Could you check a few things on this model? Use its own coordinates, in mm. A direction names the side the tool comes from. Coordinates: 2 decimals unless noted, no trailing zeros. Loops run counter-clockwise (first coordinate to the right, second up) from the corner with the lowest first, then second, coordinate; pieces in that order, holes last.
from build123d import *

# Parameters (mm, degrees)
SKETCH_2_R          = 1.5
EXTRUDE_1_DEPTH     = 52
CUT_EXTRUDE_START   = -3
SKETCH_3_R          = 19
SKETCH_3_R_2        = 1.6
CUT_EXTRUDE_1_DEPTH = 25
SKETCH_3_3_R        = 1.6
CUT_EXTRUDE_2_DEPTH = 25
SKETCH_5_R          = 17.6
CUT_EXTRUDE_3_DEPTH = 310.300460798
SKETCH_6_R          = 6.1
CUT_EXTRUDE_4_DEPTH = 3
CUT_EXTRUDE_5_REACH = 313.3
SKETCH_7_W          = 42
SKETCH_7_H          = 28
CHAMFER_1_SIZE      = 5
CHAMFER_5_SIZE      = 10
CHAMFER_5_SIZE2     = 5.773502692
EXTRUDE_2_DEPTH     = 2


with BuildPart() as part:
    # 草图2 → 凸台-拉伸1 (new body)
    with BuildSketch(Plane(origin=(0, 0, 255.313805399), x_dir=(-1, 0, 0), z_dir=(0, 0, -1))):
        Polygon((21, 18), (19, 20), (-19, 20), (-21, 18), (-21, -25), (21, -25), align=None)
        with Locations((16, -15)):
            Circle(SKETCH_2_R, mode=Mode.SUBTRACT)
        with Locations((16, 15)):
            Circle(SKETCH_2_R, mode=Mode.SUBTRACT)
        with Locations((-16, 15)):
            Circle(SKETCH_2_R, mode=Mode.SUBTRACT)
        with Locations((-16, -15)):
            Circle(SKETCH_2_R, mode=Mode.SUBTRACT)
    extrude(amount=-EXTRUDE_1_DEPTH)

    # 草图3 → 切除-拉伸1 (cut)
    # profile 1 of 7: a face of its own
    with BuildSketch(Plane.XZ.offset(25).offset(CUT_EXTRUDE_START)):
        with Locations(Location((0, 279.313805399, 0), (0, 0, 270))):
            Circle(SKETCH_3_R)
        with Locations((15.5, 279.313805399)):
            Circle(SKETCH_3_R_2, mode=Mode.SUBTRACT)
        with Locations((7.75, 292.737199157)):
            Circle(SKETCH_3_R_2, mode=Mode.SUBTRACT)
        with Locations((-7.75, 292.737199157)):
            Circle(SKETCH_3_R_2, mode=Mode.SUBTRACT)
        with Locations((-15.5, 279.313805399)):
            Circle(SKETCH_3_R_2, mode=Mode.SUBTRACT)
        with Locations((-7.75, 265.89041164)):
            Circle(SKETCH_3_R_2, mode=Mode.SUBTRACT)
        with Locations((7.75, 265.89041164)):
            Circle(SKETCH_3_R_2, mode=Mode.SUBTRACT)
    # profile 2 of 7: a face of its own
    with BuildSketch(Plane.XZ.offset(25).offset(CUT_EXTRUDE_START)):
        with Locations((7.75, 292.737199157)):
            Circle(SKETCH_3_R_2)
    # profile 3 of 7: a face of its own
    with BuildSketch(Plane.XZ.offset(25).offset(CUT_EXTRUDE_START)):
        with Locations((-7.75, 292.737199157)):
            Circle(SKETCH_3_R_2)
    # profile 4 of 7: a face of its own
    with BuildSketch(Plane.XZ.offset(25).offset(CUT_EXTRUDE_START)):
        with Locations((-15.5, 279.313805399)):
            Circle(SKETCH_3_R_2)
    # profile 5 of 7: a face of its own
    with BuildSketch(Plane.XZ.offset(25).offset(CUT_EXTRUDE_START)):
        with Locations((-7.75, 265.89041164)):
            Circle(SKETCH_3_R_2)
    # profile 6 of 7: a face of its own
    with BuildSketch(Plane.XZ.offset(25).offset(CUT_EXTRUDE_START)):
        with Locations((7.75, 265.89041164)):
            Circle(SKETCH_3_R_2)
    # profile 7 of 7: a face of its own
    with BuildSketch(Plane.XZ.offset(25).offset(CUT_EXTRUDE_START)):
        with Locations((15.5, 279.313805399)):
            Circle(SKETCH_3_R_2)
    extrude(amount=-CUT_EXTRUDE_1_DEPTH, mode=Mode.SUBTRACT)

    # 草图3<3> → 切除-拉伸2 (cut)
    with BuildSketch(Plane.XZ.offset(25)):
        with Locations(Location((-7.75, 292.737199157, 0), (0, 0, 270))):
            Circle(SKETCH_3_3_R)
        with Locations(Location((7.75, 292.737199157, 0), (0, 0, 270))):
            Circle(SKETCH_3_3_R)
        with Locations(Location((-15.5, 279.313805399, 0), (0, 0, 270))):
            Circle(SKETCH_3_3_R)
        with Locations(Location((-7.75, 265.89041164, 0), (0, 0, 270))):
            Circle(SKETCH_3_3_R)
        with Locations(Location((7.75, 265.89041164, 0), (0, 0, 270))):
            Circle(SKETCH_3_3_R)
        with Locations(Location((15.5, 279.313805399, 0), (0, 0, 270))):
            Circle(SKETCH_3_3_R)
    extrude(amount=-CUT_EXTRUDE_2_DEPTH, mode=Mode.SUBTRACT)

    # 草图5 → 切除-拉伸3 (cut, through all)
    with BuildSketch(Plane.XZ.offset(-3)):
        with Locations(Location((0, 279.313805399, 0), (0, 0, 270))):
            Circle(SKETCH_5_R)
    extrude(amount=-CUT_EXTRUDE_3_DEPTH, mode=Mode.SUBTRACT)

    # 草图6 → 切除-拉伸4 (cut)
    with BuildSketch(Plane.XZ.offset(25)):
        with Locations(Location((0, 286.313805399, 0), (0, 0, 270))):
            Circle(SKETCH_6_R)
    extrude(amount=-CUT_EXTRUDE_4_DEPTH, mode=Mode.SUBTRACT)

    # 切除-拉伸5: up to this face of the body (flat: up to its plane)
    cut_extrude_5_end = Plane(part.part.faces().sort_by_distance((0, -22, 278.469302594))[0])
    # 草图7 → 切除-拉伸5 (cut, up to the picked face)
    with BuildSketch(Plane(origin=(0, 20, 0), x_dir=(1, 0, 0), z_dir=(0, 1, 0)), mode=Mode.PRIVATE) as cut_extrude_5_sk1:
        with Locations((0, -293.313805399)):
            Rectangle(SKETCH_7_W, SKETCH_7_H)
    cut_extrude_5_tool1 = split(extrude(cut_extrude_5_sk1.sketch, amount=-CUT_EXTRUDE_5_REACH, mode=Mode.PRIVATE), bisect_by=cut_extrude_5_end, keep=Keep.BOTH, mode=Mode.PRIVATE)
    add(cut_extrude_5_tool1.solids().sort_by(Axis((0, 20, 293.313805), (0, -1, 0)))[0], mode=Mode.SUBTRACT)

    # 倒角1
    chamfer_1_edges = [part.edges().sort_by_distance(p)[0] for p in [
        (21, -23.5, 307.313805399),
        (-21, -23.5, 307.313805399),
    ]]
    chamfer(chamfer_1_edges, length=CHAMFER_1_SIZE)

    # 倒角5
    chamfer_5_edges = [part.edges().sort_by_distance(p)[0] for p in [
        (-18.3, 20, 279.313805399),
        (18.3, 20, 279.313805399),
    ]]
    chamfer_5_side = [part.faces().sort_by_distance(p)[0] for p in [
        (0, 20, 255.7632495),
    ]]
    chamfer(chamfer_5_edges, length=CHAMFER_5_SIZE, length2=CHAMFER_5_SIZE2, reference=chamfer_5_side[0])

    # 草图8 → 凸台-拉伸2 (add)
    with BuildSketch(Plane(origin=(21, 0, 0), x_dir=(0, 0, -1), z_dir=(1, 0, 0))):
        Polygon((-279.313805399, -22), (-279.313805399, 2.989978389), (-290.216930942, -22), align=None)
    extrude_2 = extrude(amount=-EXTRUDE_2_DEPTH)

    # 镜向1: 凸台-拉伸2 across plane
    add(extrude_2.mirror(Plane(origin=(0, 0, 0), x_dir=(0, 0, 1), z_dir=(1, 0, 0))))


solid = part.part
(1) Imagine slicing it at C-C, the plane y = 12.5. Write out the boundary of the cut face in (x, z), and give its area (3 significant figures).
Answers:
outline: (-21, 255.31) - (21, 255.31) - (21, 279.31) - (17.6, 279.31) arc R17.6 cw to (-17.6, 279.31) - (-21, 279.31) - close
area: 521 mm2
(2) I need wall thicknesses on probe 1 along X at (y, z) = (-12, 280.5); probe 2 along X at (y, z) = (-14, 258); probe 3 along Z at (x, y) = (-7, -23). Which ranges of each line are inside material? Lowest first, please.
Answers:
probe 1: x = -21 to -19, 19 to 21
probe 2: x = -21 to -17.12, -14.88 to 14.88, 17.12 to 21
probe 3: z = 255.31 to 264.48, 267.3 to 291.32, 294.15 to 307.31
(3) We'd pull the mould along X, two halves only. Please class faces 5 (the face through (20.01, -9.33, 284.69)), 6 (the face through (20, 19, 264)), 7 (the face through (15.57, -23.521, 280.912)): +X half, -X half, draft (parallel to the pull), parting line (faces both ways), or undercut.
Answers:
face 5: draft
face 6: +X half
face 7: undercut
(4) Imagine slicing it at D-D, the plane y = -15. Write out the boundary of the cut face in (x, z).
Answers:
outline: (-21, 255.31) - (-17.5, 255.31) - (-17.5, 271.91) arc R19 cw to (-19, 279.31) - (-19, 287.16) - (-21, 287.16) - close; (-14.5, 255.31) - (14.5, 255.31) - (14.5, 267.04) arc R19 cw to (-14.5, 267.04) - close; (17.5, 255.31) - (21, 255.31) - (21, 287.16) - (19, 287.16) - (19, 279.31) arc R19 cw to (17.5, 271.91) - close
(5) Which directions (+Z, -Z, +X, -X, +Y, -Y) give clear straight access to the entire face, cutting with the end or side of a thin tool? Please do faces 1 (the face through (0, -2, 255.314)), 2 (the face through (0, 3, 261)), 3 (the face through (19, 9, 279.314)), 4 (the face through (-19, -15, 282)).
Answers:
face 1: -Z, +X, -X, +Y, -Y
face 2: +Z
face 3: +Z, +X, -X, +Y
face 4: +Z, +Y
(6) Imagine slicing it at B-B, the plane z = 285. Write out the boundary of the cut face in (x, y), and give its area (3 significant figures).
Answers:
outline: (-21, -25) - (-5.96, -25) - (-5.96, -22) - (-19, -22) - (-19, -10.04) - (-21, -10.04) - close; (5.96, -25) - (21, -25) - (21, -10.04) - (19, -10.04) - (19, -22) - (5.96, -22) - close
area: 138 mm2
(7) Imagine slicing it at A-A, the plane x = -1. Write out the boundary of the cut face in (y, z).
Answers:
outline: (-25, 255.31) - (20, 255.31) - (20, 261.74) - (3, 261.74) - (3, 260.34) - (-22, 260.34) - (-22, 280.3) - (-25, 280.3) - close; (-25, 292.33) - (-22, 292.33) - (-22, 307.31) - (-25, 307.31) - close
(8) For pin 1 (1.8 mm diameter, centred on x = -16, y = -15, fed in from -Z); pin 2 (1.7 mm diameter, centred on x = -19.5, y = 7, fed in from +Z); pin 3 (5 mm diameter, centred on x = 15.5, z = 279.31, fed in from +Y); pin 4 (12.5 mm diameter, centred on x = 5, z = 290.5, fed in from +Y), each with a flat end and sliding along its axis, tell me the tip position at first contact or that it passes through.
Answers:
pin 1: passes through
pin 2: stops at z = 279.31
pin 3: stops at y = 15.06
pin 4: stops at y = -22
